Can you work these out from the drawing? Everything is in mm from the part's minimum corner. A direction names the side the tool comes from. Coordinates: 2 decimals unless noted, no trailing zeros. Loops run counter-clockwise (first coordinate to the right, second up) from the corner with the lowest first, then second, coordinate; pieces in that order, holes last. Notation, with made-up numbers: M -5,85.5 L 24,85.5 A29 ccw 24,124.5 Z; hole C 45.25,87.5 d3. An arc over 180 degrees is marked long. Use CSV: the item, a comma, the result in double quotes. Start each with the question number.
Q1. If we section it at A-A (y = 60): Please give me the cut outline in (x, z).
Q2. For pin 1 Ø1.5 at (x, y) = (4.5, 47) entering from +Z; pin 2 Ø12.5 at (y, z) = (85, 51) entering from +X; pin 3 Ø22 at (x, z) = (15.5, 53) entering from -Y, each with a flat end and sliding along its axis, tell me the tip position at first contact or that it passes through.
Q3. If we section it at B-B (x = 12.5): Please give me the cut outline in (y, z), and give its area (3 significant figures).
Q4. Which directions (+Z, -Z, +X, -X, +Y, -Y) give clear straight access to the entire face, cutting with the end or side of a thin tool? Please do the marked faces 1, 2, 3 and 4.
Q5. If we section it at D-D (y = 81.5): Please give me the cut outline in (x, z).
Q6. If we section it at C-C (z = 8.5): Please give me the cut outline in (x, y).
Q7. Please list where these lines run through material, in increasing order: probe 1 along Z at (x, y) = (32, 62); probe 2 along X at (y, z) = (71, 42.5); probe 3 along Y at (x, z) = (5, 33). Write a range as [from, to].
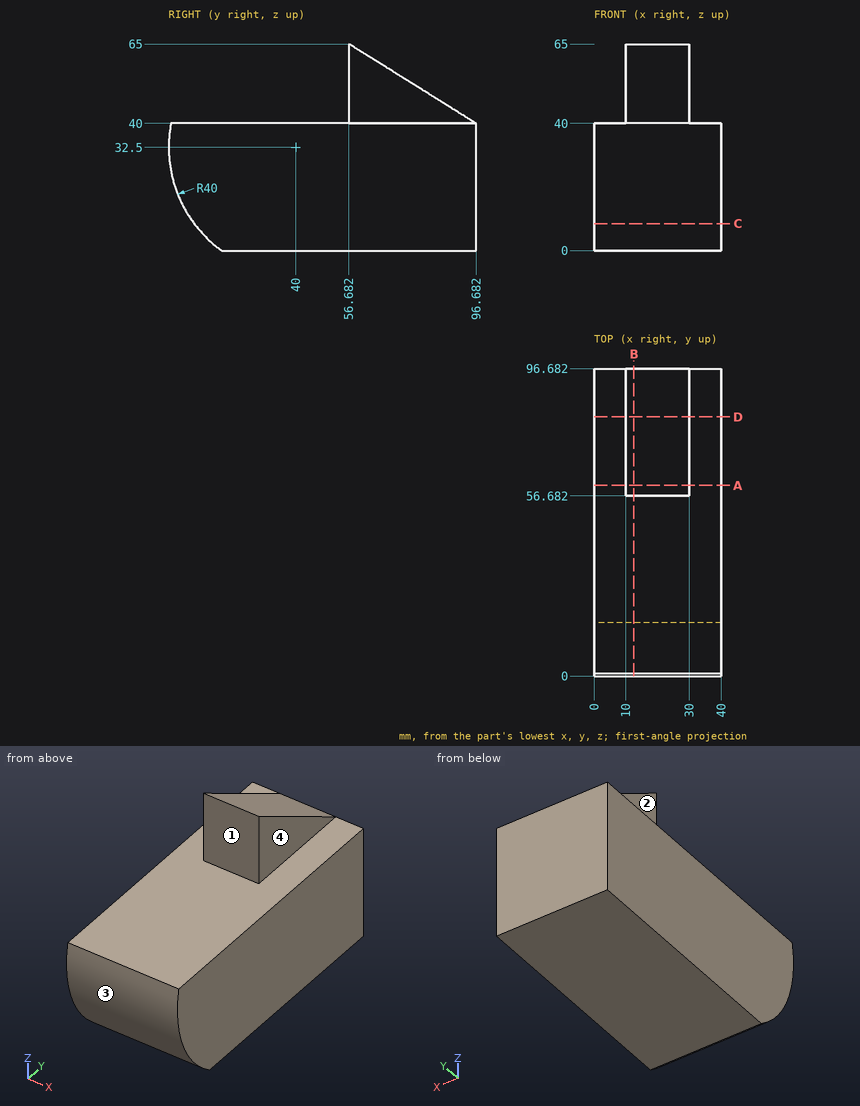
Results below:
1,outline,"M 0,0 L 40,0 L 40,40 L 30,40 L 30,62.93 L 10,62.93 L 10,40 L 0,40 Z"
2,pin 1,"z = 40"
2,pin 2,"x = 30"
2,pin 3,"y = 56.68"
3,outline,"M 0.71,40 A40 ccw 16.68,0 L 96.68,0 L 96.68,40 L 56.68,65 L 56.68,40 Z"
3,area,"4,200 mm^2"
4,face 1,"+Z, +X, -X, -Y"
4,face 2,"+Z, -X, +Y, -Y"
4,face 3,"+X, -X, -Y"
4,face 4,"+Z, +X, +Y, -Y"
5,outline,"M 0,0 L 40,0 L 40,40 L 30,40 L 30,49.49 L 10,49.49 L 10,40 L 0,40 Z"
6,outline,"M 0,8 L 40,8 L 40,96.68 L 0,96.68 Z"
7,probe 1,"[0, 40]"
7,probe 2,"[10, 30]"
7,probe 3,"[0, 96.68]"
